```python
from build123d import *
from build123d.topology import SkipClean

# Parameters (mm, degrees)
SKETCH1_R             = 24.8
SKETCH1_R_2           = 2
BOSS_EXTRUDE1_DEPTH   = 8.75
BOSS_EXTRUDE3_START   = 0.5
SKETCH3_R             = 12.5
SKETCH3_R_2           = 2
BOSS_EXTRUDE3_DEPTH   = 0.5
CUT_EXTRUDE1_DEPTH    = 1.5
CIRPATTERN1_COUNT     = 5
SKETCH5_R             = 11.7
CUT_EXTRUDE2_DEPTH    = 0.5
BOSS_EXTRUDE4_START   = 0.78
SKETCH6_R             = 3.92
SKETCH6_R_2           = 2
BOSS_EXTRUDE4_DEPTH   = 0.78
MIRROR1_START         = 7.75
MIRROR1_DEPTH         = 1
MIRROR1_START_2       = 8.75
MIRROR1_2_OUTLINE_R   = 12.5
MIRROR1_2_OUTLINE_R_2 = 11.7
MIRROR1_2_OUTLINE_R_3 = 3.92
MIRROR1_2_OUTLINE_R_4 = 2
MIRROR1_2_DEPTH       = 0.5
MIRROR1_START_3       = 9.25
MIRROR1_3_OUTLINE_R   = 3.92
MIRROR1_3_OUTLINE_R_2 = 2
MIRROR1_3_DEPTH       = 0.28


# Read off the part's stored shape, not the designer's step: Mirror1
with BuildPart() as part:
    # Sketch1 → Boss-Extrude1 (new, symmetric)
    with BuildSketch(Plane.XY):
        Circle(SKETCH1_R)
        Circle(SKETCH1_R_2, mode=Mode.SUBTRACT)
    extrude(amount=BOSS_EXTRUDE1_DEPTH, both=True)

    # Sketch3 → Boss-Extrude3 (add)
    with SkipClean():  # the faces are left unmerged after this step: merging them gives an invalid solid
        with BuildSketch(Plane(origin=(0, 0, -8.75), x_dir=(-1, 0, 0), z_dir=(0, 0, -1)).offset(BOSS_EXTRUDE3_START)):
            with Locations(Location((0, 0, 0), (0, 0, 180))):
                Circle(SKETCH3_R)
            Circle(SKETCH3_R_2, mode=Mode.SUBTRACT)
        extrude(amount=-BOSS_EXTRUDE3_DEPTH)

    # Sketch4 → Cut-Extrude1 (cut)
    with SkipClean():  # the faces are left unmerged after this step: merging them gives an invalid solid
        with BuildSketch(Plane(origin=(0, 0, -9.25), x_dir=(-1, 0, 0), z_dir=(0, 0, -1))):
            with BuildLine():
                Line((-3.088094758, 10.3), (3.088094758, 10.3))
                ThreePointArc((3.088094758, 10.3), (3.963605368, 9.783198895), (3.934186276, 8.766962344))
                Line((3.934186276, 8.766962344), (2.044186276, 5.766962344))
                ThreePointArc((2.044186276, 5.766962344), (1.681293653, 5.42448939), (1.198094758, 5.3))
                Line((1.198094758, 5.3), (-1.198094758, 5.3))
                ThreePointArc((-1.198094758, 5.3), (-1.681293653, 5.42448939), (-2.044186276, 5.766962344))
                Line((-2.044186276, 5.766962344), (-3.934186276, 8.766962344))
                ThreePointArc((-3.934186276, 8.766962344), (-3.963605368, 9.783198895), (-3.088094758, 10.3))
            make_face()
        cut_extrude1 = extrude(amount=-CUT_EXTRUDE1_DEPTH, mode=Mode.SUBTRACT)

    # CirPattern1: Cut-Extrude1 ×5 about axis
    with SkipClean():  # the faces are left unmerged after this step: merging them gives an invalid solid
        cirpattern1_axis = Axis((0, 0, 0), (0, 0, 1))
        for i in range(1, CIRPATTERN1_COUNT):
            add(cut_extrude1.rotate(cirpattern1_axis, i * 360 / CIRPATTERN1_COUNT), mode=Mode.SUBTRACT)

    # Sketch5 → Cut-Extrude2 (cut)
    with BuildSketch(Plane(origin=(0, 0, -9.25), x_dir=(-1, 0, 0), z_dir=(0, 0, -1))):
        Circle(SKETCH5_R)
    extrude(amount=-CUT_EXTRUDE2_DEPTH, mode=Mode.SUBTRACT)

    # Sketch6 → Boss-Extrude4 (add)
    with BuildSketch(Plane(origin=(0, 0, -8.75), x_dir=(-1, 0, 0), z_dir=(0, 0, -1)).offset(BOSS_EXTRUDE4_START)):
        with Locations(Location((0, 0, 0), (0, 0, 180))):
            Circle(SKETCH6_R)
        Circle(SKETCH6_R_2, mode=Mode.SUBTRACT)
    extrude(amount=-BOSS_EXTRUDE4_DEPTH)

    # Mirror1 outline → Mirror1 (cut)
    with BuildSketch(Plane.XY.offset(MIRROR1_START)):
        with BuildLine():
            Line((-1.970267616, -9.405078198), (-1.735953979, -5.867113088))
            ThreePointArc((-1.735953979, -5.867113088), (-1.828239727, -5.376743716), (-2.145982817, -4.9920125))
            Line((-2.145982817, -4.9920125), (-4.084540858, -3.58356764))
            ThreePointArc((-4.084540858, -3.58356764), (-4.548630003, -3.400264488), (-5.043516853, -3.464027996))
            Line((-5.043516853, -3.464027996), (-8.33591473, -4.780164852))
            ThreePointArc((-8.33591473, -4.780164852), (-8.957044133, -5.585025384), (-8.552509238, -6.517738485))
            Line((-8.552509238, -6.517738485), (-3.555866959, -10.148011599))
            ThreePointArc((-3.555866959, -10.148011599), (-2.543795928, -10.244522947), (-1.970267616, -9.405078198))
        make_face()
        with BuildLine():
            Line((8.33591473, -4.780164852), (5.043516853, -3.464027996))
            ThreePointArc((5.043516853, -3.464027996), (4.548630003, -3.400264488), (4.084540858, -3.58356764))
            Line((4.084540858, -3.58356764), (2.145982817, -4.9920125))
            ThreePointArc((2.145982817, -4.9920125), (1.828239727, -5.376743716), (1.735953979, -5.867113088))
            Line((1.735953979, -5.867113088), (1.970267616, -9.405078198))
            ThreePointArc((1.970267616, -9.405078198), (2.543795928, -10.244522947), (3.555866959, -10.148011599))
            Line((3.555866959, -10.148011599), (8.552509238, -6.517738485))
            ThreePointArc((8.552509238, -6.517738485), (8.957044133, -5.585025384), (8.33591473, -4.780164852))
        make_face()
        with BuildLine():
            Line((7.122146247, 6.450773848), (4.853018817, 3.726226049))
            ThreePointArc((4.853018817, 3.726226049), (4.639447671, 3.275264692), (4.670367895, 2.777245897))
            Line((4.670367895, 2.777245897), (5.410831178, 0.498334243))
            ThreePointArc((5.410831178, 0.498334243), (5.678544293, 0.077254123), (6.116395415, -0.162047309))
            Line((6.116395415, -0.162047309), (9.553607084, -1.032493141))
            ThreePointArc((9.553607084, -1.032493141), (10.529196477, -0.746437996), (10.750155878, 0.245922399))
            Line((10.750155878, 0.245922399), (8.841608357, 6.119827685))
            ThreePointArc((8.841608357, 6.119827685), (8.079553641, 6.792787431), (7.122146247, 6.450773848))
        make_face()
        with BuildLine():
            Line((-3.934186276, 8.766962344), (-2.044186276, 5.766962344))
            ThreePointArc((-2.044186276, 5.766962344), (-1.681293653, 5.42448939), (-1.198094758, 5.3))
            Line((-1.198094758, 5.3), (1.198094758, 5.3))
            ThreePointArc((1.198094758, 5.3), (1.681293653, 5.42448939), (2.044186276, 5.766962344))
            Line((2.044186276, 5.766962344), (3.934186276, 8.766962344))
            ThreePointArc((3.934186276, 8.766962344), (3.963605368, 9.783198895), (3.088094758, 10.3))
            Line((3.088094758, 10.3), (-3.088094758, 10.3))
            ThreePointArc((-3.088094758, 10.3), (-3.963605368, 9.783198895), (-3.934186276, 8.766962344))
        make_face()
        with BuildLine():
            Line((-9.553607084, -1.032493141), (-6.116395415, -0.162047309))
            ThreePointArc((-6.116395415, -0.162047309), (-5.678544293, 0.077254123), (-5.410831178, 0.498334243))
            Line((-5.410831178, 0.498334243), (-4.670367895, 2.777245897))
            ThreePointArc((-4.670367895, 2.777245897), (-4.639447671, 3.275264692), (-4.853018817, 3.726226049))
            Line((-4.853018817, 3.726226049), (-7.122146247, 6.450773848))
            ThreePointArc((-7.122146247, 6.450773848), (-8.079553641, 6.792787431), (-8.841608357, 6.119827685))
            Line((-8.841608357, 6.119827685), (-10.750155878, 0.245922399))
            ThreePointArc((-10.750155878, 0.245922399), (-10.529196477, -0.746437996), (-9.553607084, -1.032493141))
        make_face()
    extrude(amount=MIRROR1_DEPTH, mode=Mode.SUBTRACT)

    # Mirror1 2 outline → Mirror1 2 (add)
    # profile 1 of 2: a face of its own
    with BuildSketch(Plane.XY.offset(MIRROR1_START_2)):
        Circle(MIRROR1_2_OUTLINE_R)
        Circle(MIRROR1_2_OUTLINE_R_2, mode=Mode.SUBTRACT)
    # profile 2 of 2: a face of its own
    with BuildSketch(Plane.XY.offset(MIRROR1_START_2)):
        Circle(MIRROR1_2_OUTLINE_R_3)
        Circle(MIRROR1_2_OUTLINE_R_4, mode=Mode.SUBTRACT)
    extrude(amount=MIRROR1_2_DEPTH)

    # Mirror1 3 outline → Mirror1 3 (add)
    with BuildSketch(Plane.XY.offset(MIRROR1_START_3)):
        Circle(MIRROR1_3_OUTLINE_R)
        Circle(MIRROR1_3_OUTLINE_R_2, mode=Mode.SUBTRACT)
    extrude(amount=MIRROR1_3_DEPTH)


solid = part.part
```
The model under review builds one solid part; all positions refer to its coordinate system, in mm. A direction names the side the tool comes from. Coordinates: 2 decimals unless noted, no trailing zeros. Write each loop counter-clockwise with the first axis right and the second up, starting at its lowest first coordinate (ties: lowest second). Pieces come first, ordered by that corner, then holes. Notation, with made-up numbers: (68.25, 10.25) -> (94.25, 10.25) arc R17 cw to (94.25, 36.25) -> close; hole circle Ø9 at (-26.5, 68). An arc over 180 degrees is marked (long way). One line per item, written item: value. Start each with the question number.
Q1. Add section B-B, the plane x = -13.5. Give the boundary of the cut face in (y, z).
Q2. For faces 1 (the face through (-2, 1, 9.53)), 2 (the face through (11.923, -3.755, -9.004)), 3 (the face through (-6.667, -4.113, 8.243)), list the 3-axis set-ups (+Z, -Z, +X, -X, +Y, -Y) from which the entire face can be reached by the end or side of a thin tool; tool diameter is ignored.
Q3. The part is to be moulded in two halves that separate along Y. For faces 4 (the face through (-3.002, 7.288, 8.243)), 5 (the face through (-5.9, 11.4, -8.75)), 6 (the face through (11.444, -22.002, 0.123)), say which applies: +Y half, -Y half, draft (parallel to the pull), parting line (faces both ways), or undercut.
Q4. Clearance check with flat-ended pins moving along their axes: P1, Ø3, axis at x = -17.5, y = -19.5, coming from the +Z side; P2, Ø0.8, axis at x = -0.5, z = -8.5, coming from the -Y side; P3, Ø1, axis at y = -3.5, z = -7, coming from the -X side. State where each tip first meets the part, or that it passes through.
Q5. To check wall thickness, follow probe 1 along Y at (x, z) = (0, 9.4); probe 2 along X at (y, z) = (4.5, 8.25); probe 3 along Z at (x, y) = (3.5, 5). State the ranges of each line that lie inside material, in increasing order.
Q6. Add section A-A, the plane z = 2.25. Give the boundary of the cut face in (x, y).
Response:
1. outline: (-20.8, -8.75) -> (20.8, -8.75) -> (20.8, 8.75) -> (-20.8, 8.75) -> close
2. face 1: +Z, +X, -X, +Y, -Y
2. face 2: -Z
2. face 3: +Z
3. face 4: undercut
3. face 5: draft
3. face 6: parting line
4. P1: z = 8.75
4. P2: y = -24.8
4. P3: x = -24.62
5. probe 1: -3.92 to -2, 2 to 3.92
5. probe 2: -24.39 to -9.37, -5.5 to 5.5, 9.37 to 24.39
5. probe 3: -8.75 to 8.75
6. outline: circle Ø49.6 at (0, 0); hole circle Ø4 at (0, 0)
